from build123d import *

# Parameters (mm, degrees)
F1_DEPTH = 9
F2_W     = 180
F2_H     = 120
F2_W_2   = 160
F3_DEPTH = 25


with BuildPart() as f1:
    # F0 (on Right) → F1 (new body)
    with BuildSketch(Plane.YZ):
        Polygon((0, 296), (0, 0), (321, 0), (321, 630), (-169, 630), (-169, 316), (-149, 296), align=None)
    extrude(amount=F1_DEPTH)

    # F2 (on face) → F3 (cut)
    with BuildSketch(Plane(origin=(0, 0, 0), x_dir=(0, -1, 0), z_dir=(-1, 0, 0))):
        with Locations((-201, 366)):
            Rectangle(F2_W, F2_H)
        with Locations((-211, 90)):
            Rectangle(F2_W_2, F2_H)
    extrude(amount=-F3_DEPTH, mode=Mode.SUBTRACT)


solid = f1.part
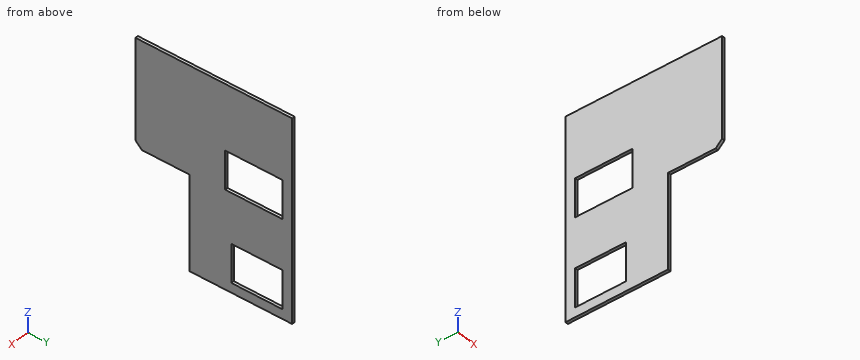
Model file for the job. Use its own axes, mm. Give positions to 0.01 mm unless a question says otherwise; leave off trailing zeros. Order: outer loops, then holes, each group sorted by start corner. A loop starts at its lowest first (then second) coordinate and runs counter-clockwise, first axis right, second up. Notation, with made-up numbers: M -14.5,-12.75 L 16.5,-12.75 A18 ccw 16.5,6.25 Z; hole C -34.75,23 d7. An arc over 180 degrees is marked long. Put each result on its own line as item: value. Start each with the question number.
(1) Band-saw the part on A-A on z = 376.5. Give the cut face in (x, y), then the cut area to 3 significant figures.
(2) Band-saw the part on B-B on x = 4.5. Give the cut face in (y, z).
(3) Pin check, flat tips, straight feed: pin 1 Ø2 at (y, z) = (56.5, 255) entering from -X; pin 2 Ø5 at (x, y) = (7, -103) entering from -Z; pin 3 Ø2.5 at (x, z) = (4.5, 159) entering from -Y. Stop position of each tip, or through.
(4) Band-saw the part on C-C on y = 197. Give the cut face in (x, z), then the cut area to 3 significant figures.
(5) Band-saw the part on D-D on z = 43. Give the cut face in (x, y), then the cut area to 3 significant figures.
(6) Drill centre lines: L1, parallel to Z at x = 4, y = 157; L2, parallel to Y at x = 0.5, z = 344; L3, parallel to Z at x = 1.5, y = 112. Where is each one in solid material? Low to high. Write a range as [from, to].
Results below:
1. outline: M 0,-169 L 9,-169 L 9,111 L 0,111 Z; M 0,291 L 9,291 L 9,321 L 0,321 Z
1. area: 2,790 mm2
2. outline: M -169,316 L -149,296 L 0,296 L 0,0 L 321,0 L 321,630 L -169,630 Z; hole M 111,306 L 291,306 L 291,426 L 111,426 Z; hole M 131,30 L 291,30 L 291,150 L 131,150 Z
3. pin 1: stops at x = 0
3. pin 2: stops at z = 296
3. pin 3: stops at y = 0
4. outline: M 0,0 L 9,0 L 9,30 L 0,30 Z; M 0,150 L 9,150 L 9,306 L 0,306 Z; M 0,426 L 9,426 L 9,630 L 0,630 Z
4. area: 3,510 mm2
5. outline: M 0,0 L 9,0 L 9,131 L 0,131 Z; M 0,291 L 9,291 L 9,321 L 0,321 Z
5. area: 1,450 mm2
6. L1: z = [0, 30], [150, 306], [426, 630]
6. L2: y = [-169, 111], [291, 321]
6. L3: z = [0, 306], [426, 630]
